Work out the finished part from the listing and answer in its coordinate system (mm). A direction names the side the tool comes from. Give positions to 0.01 mm unless a question says otherwise; leave off trailing zeros. Order: outer loops, then holes, each group sorted by start corner. A loop starts at its lowest first (then second) coordinate and runs counter-clockwise, first axis right, second up. Notation, with made-up numbers: (27, 8.25) - (81, 8.25) arc R29 ccw to (81, 35.25) - close; hole circle Ø6 at (-4, 55.25). An arc over 180 degrees is marked (long way). Write each question's results on one line, items separated by ' | '.
from build123d import *

# Parameters (mm, degrees)
SKETCH1_W           = 44
SKETCH1_H           = 54.6
SKETCH1_R           = 1
BOSS_EXTRUDE1_DEPTH = 3
SKETCH2_W           = 3
SKETCH2_H           = 3.011475899
SKETCH2_H_2         = 9
SKETCH2_H_3         = 5.958851055
CUT_EXTRUDE2_DEPTH  = 10


with BuildPart() as part:
    # Sketch1 → Boss-Extrude1 (new body)
    with BuildSketch(Plane(origin=(0, 0, 0), x_dir=(1, 0, 0), z_dir=(0, 1, 0))):
        Rectangle(SKETCH1_W, SKETCH1_H)
        with Locations(Location((2.636984901, 24.7, 0), (0, 0, 270))):
            Circle(SKETCH1_R, mode=Mode.SUBTRACT)
        with Locations(Location((6.15, 24.7, 0), (0, 0, 270))):
            Circle(SKETCH1_R, mode=Mode.SUBTRACT)
    extrude(amount=BOSS_EXTRUDE1_DEPTH)

    # Sketch2 → Cut-Extrude2 (cut)
    with BuildSketch(Plane.XZ):
        with Locations((20.5, -16.164589005)):
            Rectangle(SKETCH2_W, SKETCH2_H)
        with Locations((20.5, -4.158851055)):
            Rectangle(SKETCH2_W, SKETCH2_H_2)
        with Locations((20.5, 10.841148945)):
            Rectangle(SKETCH2_W, SKETCH2_H_2)
        with Locations((20.5, 24.320574472)):
            Rectangle(SKETCH2_W, SKETCH2_H_3)
    extrude(amount=-CUT_EXTRUDE2_DEPTH, mode=Mode.SUBTRACT)


solid = part.part
1. Determine the mould class of faces 1 (the face through (22, 1, 18)), 2 (the face through (0, 1, -27.3)), 3 (the face through (20, 1, -17.67)) for opening direction Z: +Z half, -Z half, draft (parallel to the pull), parting line (faces both ways), or undercut.
Answer list:
face 1: draft | face 2: -Z half | face 3: undercut
2. A tool of negligible diameter and unlimited length cuts with its end or side. For faces 4 (the face through (22, 1, 3)), 5 (the face through (19, 1, 24)), 6 (the face through (20, 1, -14.659)), from which of +Z, -Z, +X, -X, +Y, -Y can it reach the whole face along a straight path? Write none if from no direction.
Answer list:
face 4: +Z, -Z, +X, +Y, -Y | face 5: +Z, +X, +Y, -Y | face 6: +X, +Y, -Y
3. A cutting plane is placed at A-A, the plane z = -24.7. Write down the section's boundary in (x, y).
Answer list:
outline: (-22, 0) - (1.64, 0) - (1.64, 3) - (-22, 3) - close; (3.64, 0) - (5.15, 0) - (5.15, 3) - (3.64, 3) - close; (7.15, 0) - (22, 0) - (22, 3) - (7.15, 3) - close
4. A cutting plane is placed at C-C, the plane y = 1.75. Write down the section's boundary in (x, z), then the cut area to 3 significant figures.
Answer list:
outline: (-22, -27.3) - (22, -27.3) - (22, -17.67) - (19, -17.67) - (19, -14.66) - (22, -14.66) - (22, -8.66) - (19, -8.66) - (19, 0.34) - (22, 0.34) - (22, 6.34) - (19, 6.34) - (19, 15.34) - (22, 15.34) - (22, 21.34) - (19, 21.34) - (19, 27.3) - (-22, 27.3) - close; hole circle Ø2 at (2.64, -24.7); hole circle Ø2 at (6.15, -24.7) | area: 2,320 mm^2
5. A cutting plane is placed at D-D, the plane z = 11. Write down the section's boundary in (x, y), then the cut area to 3 significant figures.
Answer list:
outline: (-22, 0) - (19, 0) - (19, 3) - (-22, 3) - close | area: 123 mm^2
6. Given P1, Ø0.9, axis at x = 20, y = 1, coming from the +Z side; P2, Ø1.5, axis at y = 1, z = -4.5, coming from the +X side, each flat-ended and moving along its own axis, determine where each tip first touches the part or whether it passes through.
Answer list:
P1: z = 21.34 | P2: x = 19
7. A cutting plane is placed at B-B, the plane x = 6.15. Write down the section's boundary in (y, z).
Answer list:
outline: (0, -27.3) - (3, -27.3) - (3, -25.7) - (0, -25.7) - close; (0, -23.7) - (3, -23.7) - (3, 27.3) - (0, 27.3) - close
8. Straight lines are drawn through the part: line 1 (X direction, y = 0.6, z = -24.7); line 2 (Z direction, x = 6, y = 0.9); line 3 (X direction, y = 1, z = -15). For each, find the intervals that lie inside material, in ascending order. Write a range as [from, to].
Answer list:
line 1: [-22, 1.64], [3.64, 5.15], [7.15, 22] | line 2: [-27.3, -25.69], [-23.71, 27.3] | line 3: [-22, 19]
